Check sheet for the modelled part. Datum: model origin and axes. Units: mm. Face numbers are marked on the shaded views. Round coordinates to 2 decimals unless told otherwise and drop trailing zeros. Write each loop counter-clockwise with the first axis right and the second up, starting at its lowest first coordinate (ties: lowest second). Pieces come first, ordered by that corner, then holes. Notation, with made-up numbers: M 24,75 L 80,75 A26 cw 80,107 Z; hole C 80,45 d1. An arc over 180 degrees is marked long. Answer in a Markdown table with one row per item.
```python
from build123d import *

# Parameters (mm, degrees)
SKETCH001_R  = 4
HOLE_DEPTH   = 7.5
CHAMFER_SIZE = 1


with BuildPart() as part:
    # Sketch → Revolution (revolve)
    with BuildSketch(Plane.YZ):
        Polygon((2, 0), (9.7, 0), (9.25, 9), (7, 22.8), (2, 22.8), align=None)
    revolve(axis=Axis((0, 0, 0), (0, 0, 1)))

    # Sketch001 (on Face4 of Revolution) → Hole (cut)
    with BuildSketch(Plane(origin=(0, 0, 22.8), x_dir=(0, -1, 0), z_dir=(0, 0, 1))):
        Circle(SKETCH001_R)
    extrude(amount=-HOLE_DEPTH, mode=Mode.SUBTRACT)

    # Chamfer
    chamfer_edges = [part.edges().sort_by_distance(p)[0] for p in [
        (0, -9.7, 0),
    ]]
    chamfer(chamfer_edges, length=CHAMFER_SIZE)


solid = part.part
```
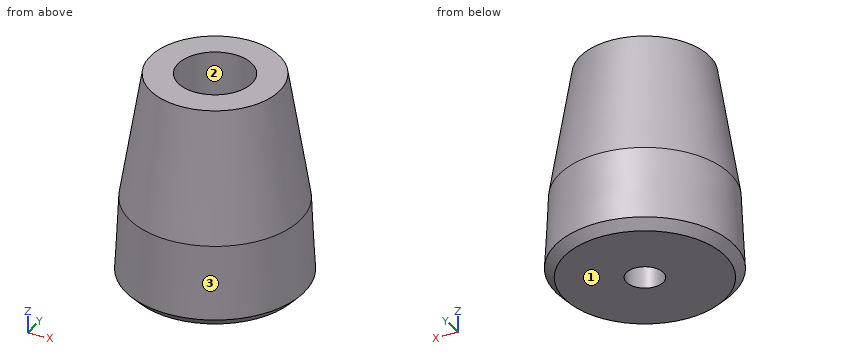
1. Section check D-D, the plane z = 7. Record the cut outline in (x, y), and give its area (3 significant figures).
Found:
| item | result |
|---|---|
| outline | C 0,0 d18.7; hole C 0,0 d4 |
| area | 262 mm2 |
2. Go/stop test with flat-tipped pins: pin 1 (4 mm diameter, centred on x = 1.5, y = 0.5, fed in from +Z); pin 2 (8 mm diameter, centred on x = -1.5, z = 13, fed in from +Y); pin 3 (10 mm diameter, centred on x = 2.5, z = 13.5, fed in from -Y). Record where each tip stops, or that it passes through.
Found:
| item | result |
|---|---|
| pin 1 | stops at z = 15.3 |
| pin 2 | stops at y = 9.22 |
| pin 3 | stops at y = -9.24 |
3. Scan lines: L1, parallel to X at y = -1, z = 21.5; L2, parallel to X at y = -1.5, z = 17; L3, parallel to Y at x = 0, z = 5. Record each from-to range of solid material in increasing order.
Found:
| item | result |
|---|---|
| L1 | x = -7.14 to -3.87, 3.87 to 7.14 |
| L2 | x = -7.8 to -3.71, 3.71 to 7.8 |
| L3 | y = -9.45 to -2, 2 to 9.45 |
4. Section check C-C, the plane z = 2. Record the cut outline in (x, y).
Found:
| item | result |
|---|---|
| outline | C 0,0 d19.2; hole C 0,0 d4 |
5. Draft check along X on the marked faces 1, 2 and 3. Enter one of: +X half, -X half, draft (parallel to the pull), parting line (faces both ways), or undercut.
Found:
| item | result |
|---|---|
| face 1 | draft |
| face 2 | undercut |
| face 3 | parting line |
6. Section check A-A, the plane y = 0. Record the cut outline in (x, z).
Found:
| item | result |
|---|---|
| outline | M -9.65,1 L -8.7,0 L -2,0 L -2,15.3 L -4,15.3 L -4,22.8 L -7,22.8 L -9.25,9 Z; M 2,0 L 8.7,0 L 9.65,1 L 9.25,9 L 7,22.8 L 4,22.8 L 4,15.3 L 2,15.3 Z |
